Build history of the part. All positions in model axes, mm. Round coordinates to 2 decimals unless told otherwise and drop trailing zeros. Order: outer loops, then holes, each group sorted by start corner. A loop starts at its lowest first (then second) coordinate and runs counter-clockwise, first axis right, second up. Notation, with made-up numbers: (62.5, 68) -> (100.5, 68) arc R10 ccw to (100.5, 75) -> close; hole circle Ø7 at (-39, 87). An arc over 180 degrees is marked (long way). Answer as a JSON object with one key per item and string values.
from build123d import *

# Parameters (mm, degrees)
SKETCH1_R           = 2.15
BOSS_EXTRUDE1_DEPTH = 3.175
SKETCH3_R           = 2.15
BOSS_EXTRUDE3_DEPTH = 3.175
BOSS_EXTRUDE4_DEPTH = 3.175
FILLET1_R           = 6
SKETCH5_R           = 7
CUT_EXTRUDE1_DEPTH  = 10
SKETCH6_R           = 1.65
CUT_EXTRUDE2_DEPTH  = 10
SKETCH7_R           = 2.15
CUT_EXTRUDE3_DEPTH  = 10
SKETCH8_R           = 2.15
CUT_EXTRUDE4_DEPTH  = 170.219031509


with BuildPart() as part:
    # Sketch1 → Boss-Extrude1 (new body)
    with BuildSketch(Plane.XY):
        Polygon((-40, 70), (-55, 70), (-55, -70), (55, -70), (55, 70), (40, 70), (40, 35), (-40, 35), align=None)
        with Locations((-27, -52)):
            Circle(SKETCH1_R, mode=Mode.SUBTRACT)
        with Locations((27, -52)):
            Circle(SKETCH1_R, mode=Mode.SUBTRACT)
        with Locations((-27, 20)):
            Circle(SKETCH1_R, mode=Mode.SUBTRACT)
        with Locations((-47.5, 40)):
            Circle(SKETCH1_R, mode=Mode.SUBTRACT)
        with Locations((-47.5, 60)):
            Circle(SKETCH1_R, mode=Mode.SUBTRACT)
        with Locations((27, 20)):
            Circle(SKETCH1_R, mode=Mode.SUBTRACT)
        with Locations((47.5, 40)):
            Circle(SKETCH1_R, mode=Mode.SUBTRACT)
        with Locations((47.5, 60)):
            Circle(SKETCH1_R, mode=Mode.SUBTRACT)
    extrude(amount=BOSS_EXTRUDE1_DEPTH)

    # Sketch3 → Boss-Extrude3 (add)
    # profile 1 of 2: a face of its own
    with BuildSketch(Plane.XY.offset(3.175)):
        with BuildLine():
            ThreePointArc((-55, 26.72135955), (-95, -18), (-55, -62.72135955))
            Line((-55, -62.72135955), (-55, 26.72135955))
        make_face()
        with Locations((-68.75, -50.475952642)):
            Circle(SKETCH3_R, mode=Mode.SUBTRACT)
        with Locations((-87.5, -18)):
            Circle(SKETCH3_R, mode=Mode.SUBTRACT)
        with Locations((-68.75, 14.475952642)):
            Circle(SKETCH3_R, mode=Mode.SUBTRACT)
    # profile 2 of 2: a face of its own
    with BuildSketch(Plane.XY.offset(3.175)):
        with BuildLine():
            Line((55, 26.72135955), (55, -62.72135955))
            ThreePointArc((55, -62.72135955), (95, -18), (55, 26.72135955))
        make_face()
        with Locations((68.75, -50.475952642)):
            Circle(SKETCH3_R, mode=Mode.SUBTRACT)
        with Locations((87.5, -18)):
            Circle(SKETCH3_R, mode=Mode.SUBTRACT)
        with Locations((68.75, 14.475952642)):
            Circle(SKETCH3_R, mode=Mode.SUBTRACT)
    extrude(amount=-BOSS_EXTRUDE3_DEPTH)

    # Sketch4 → Boss-Extrude4 (add)
    with BuildSketch(Plane.XY.offset(3.175)):
        with BuildLine():
            Line((-79.012371244, -52.398870836), (-70, -60))
            Line((-70, -60), (-70, -140))
            Line((-70, -140), (65, -140))
            Line((65, -140), (65, -60))
            Line((65, -60), (-38.978750739, -60))
            Line((-38.978750739, -60), (-37.516030877, -61.233673392))
            ThreePointArc((-37.516030877, -61.233673392), (-59.370723196, -62.013515501), (-79.012371244, -52.398870836))
        make_face()
    boss_extrude4 = extrude(amount=-BOSS_EXTRUDE4_DEPTH)

    # Mirror2: Boss-Extrude4 across plane
    add(boss_extrude4.mirror(Plane(origin=(0, 0, 0), x_dir=(0, 0, 1), z_dir=(1, 0, 0))))

    # Fillet1
    fillet1_edges = [part.edges().sort_by_distance(p)[0] for p in [
        (-40, 35, 1.5875),
        (40, 35, 1.5875),
        (-55, 26.72135955, 1.5875),
        (55, 26.72135955, 1.5875),
    ]]
    fillet(fillet1_edges, radius=FILLET1_R)

    # Sketch5 → Cut-Extrude1 (cut)
    with BuildSketch(Plane.XY.offset(3.175)):
        with Locations((-50, -18)):
            Circle(SKETCH5_R)
        with Locations((50, -18)):
            Circle(SKETCH5_R)
    extrude(amount=-CUT_EXTRUDE1_DEPTH, mode=Mode.SUBTRACT)

    # Sketch6 → Cut-Extrude2 (cut)
    with BuildSketch(Plane.XY.offset(3.175)):
        with Locations((-17.94, -110.5)):
            Circle(SKETCH6_R)
        with Locations((-17.94, -74.5)):
            Circle(SKETCH6_R)
        with Locations((18.06, -74.5)):
            Circle(SKETCH6_R)
        with Locations((18.06, -110.5)):
            Circle(SKETCH6_R)
    extrude(amount=-CUT_EXTRUDE2_DEPTH, mode=Mode.SUBTRACT)

    # Sketch7 → Cut-Extrude3 (cut)
    with BuildSketch(Plane.XY.offset(3.175)):
        with Locations((-55, 18)):
            Circle(SKETCH7_R)
        with Locations((55, 18)):
            Circle(SKETCH7_R)
        with Locations((55, -112)):
            Circle(SKETCH7_R)
        with Locations((-55, -112)):
            Circle(SKETCH7_R)
    extrude(amount=-CUT_EXTRUDE3_DEPTH, mode=Mode.SUBTRACT)

    # Sketch8 → Cut-Extrude4 (cut, through all)
    with BuildSketch(Plane.XY.offset(3.175)):
        with Locations((-59.2, -68)):
            Circle(SKETCH8_R)
        with Locations(Location((-59.2, -132, 0), (0, 0, 180))):
            Circle(SKETCH8_R)
        with Locations((59.2, -132)):
            Circle(SKETCH8_R)
        with Locations(Location((59.2, -68, 0), (0, 0, 180))):
            Circle(SKETCH8_R)
    extrude(amount=-CUT_EXTRUDE4_DEPTH, mode=Mode.SUBTRACT)


solid = part.part
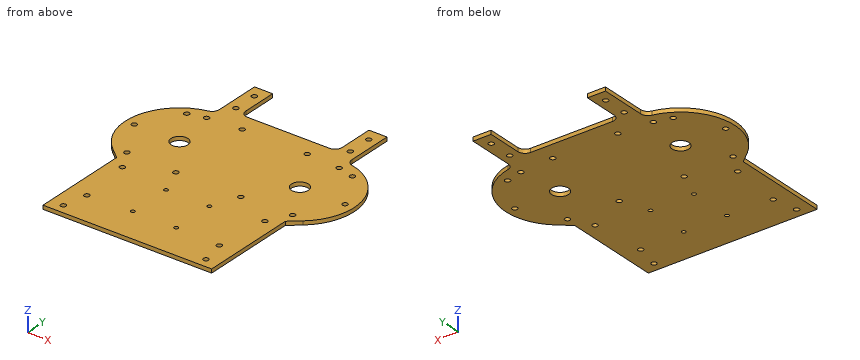
1) Cut at D-D, the plane y = -63. Give the cut face in (x, z) (3 decimals), plus the area to 4 significant figures.
Checked values:
{"outline": "(-70, 0) -> (70, 0) -> (70, 3.175) -> (-70, 3.175) -> close", "area": "444.5 mm²"}
2) Probe L1, parallel to Y at x = -27, z = 2.2; L2, parallel to X at y = -132, z = 2.2; L3, parallel to X at y = 56.5, z = 1.4. List the from-to ranges inside material, lowest first. Write a range as from..to.
Checked values:
{"L1": "y = -140..-54.15, -49.85..17.85, 22.15..35", "L2": "x = -70..-61.35, -57.05..57.05, 61.35..70", "L3": "x = -55..-40, 40..55"}
3) Flat gauge pins, fed straight in: pin 1 Ø1 at (y, z) = (62.5, 2) entering from -X; pin 2 Ø3.5 at (x, y) = (87.5, -18) entering from +Z; pin 3 Ø1.5 at (y, z) = (-45.5, 0.5) entering from +X. Where does each tip first touch, or does it go through?
Checked values:
{"pin 1": "stops at x = -55", "pin 2": "passes through", "pin 3": "stops at x = 86.19"}
4) Cut at C-C, the plane z = 2.5. Count the separate pieces of the cut face and the enclosed holes in it, plus the area to 3 significant figures.
Checked values:
{"separate pieces": "1", "enclosed holes": "28", "area": "27,500 mm²"}
5) Cut at A-A, the plane y = 54. Give the cut face in (x, z) (3 decimals), plus the area to 4 significant figures.
Checked values:
{"outline": "(-55, 0) -> (-40, 0) -> (-40, 3.175) -> (-55, 3.175) -> close; (40, 0) -> (55, 0) -> (55, 3.175) -> (40, 3.175) -> close", "area": "95.25 mm²"}
6) Cut at B-B, the plane x = -10. Give the cut face in (y, z) (3 decimals), plus the area to 3 significant figures.
Checked values:
{"outline": "(-140, 0) -> (35, 0) -> (35, 3.175) -> (-140, 3.175) -> close", "area": "556 mm²"}
